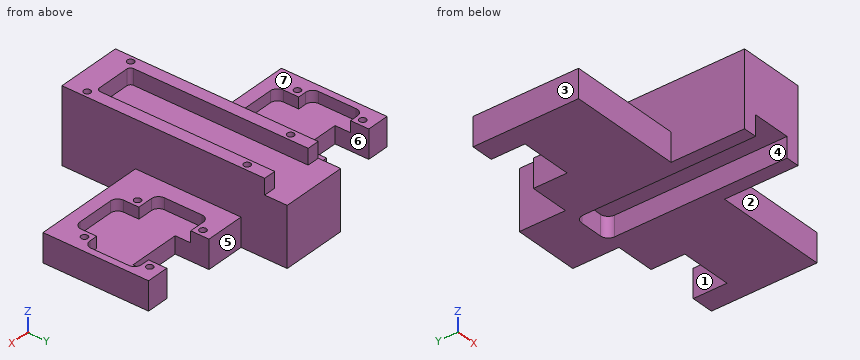
```python
from build123d import *

# Parameters (mm, degrees)
SKETCH1_W           = 130
SKETCH1_H           = 104.86
BOSS_EXTRUDE1_DEPTH = 39.84
SKETCH2_W           = 130
SKETCH2_H           = 94.86
CUT_EXTRUDE1_DEPTH  = 6.6
SKETCH3_W           = 18.25
SKETCH3_H           = 89.15
CUT_EXTRUDE2_DEPTH  = 6.98
SKETCH5_W           = 50.415
SKETCH5_H           = 94.86
CUT_EXTRUDE3_DEPTH  = 20.6
SKETCH6_R           = 1.5
CUT_EXTRUDE4_DEPTH  = 12.4
SKETCH7_W           = 50.415
SKETCH7_H           = 20.5
CUT_EXTRUDE5_DEPTH  = 12.4
SKETCH9_W           = 23
SKETCH9_H           = 15
CUT_EXTRUDE7_DEPTH  = 12.4
CUT_EXTRUDE8_DEPTH  = 5
SKETCH11_R          = 1.5
CUT_EXTRUDE9_DEPTH  = 15
FILLET2_R           = 3.175
FILLET3_R           = 3.175
FILLET4_R           = 3.175
FILLET5_R           = 1.5875
FILLET6_R           = 3.175
SKETCH12_W          = 50.415
SKETCH12_H          = 20.5
SKETCH12_W_2        = 23
SKETCH12_H_2        = 15
SKETCH12_H_3        = 27.5
SKETCH12_W_3        = 29.17
SKETCH12_H_4        = 4.86
CUT_EXTRUDE11_DEPTH = 42
SKETCH13_W          = 6.6
SKETCH13_H          = 5.14
CUT_EXTRUDE12_DEPTH = 80.585
SKETCH14_W          = 29.17
SKETCH14_H          = 10
CUT_EXTRUDE14_DEPTH = 6.98
CUT_EXTRUDE15_DEPTH = 9


with BuildPart() as part:
    # Sketch1 → Boss-Extrude1 (new body)
    with BuildSketch(Plane.XY):
        with Locations((65, -52.43)):
            Rectangle(SKETCH1_W, SKETCH1_H)
    extrude(amount=BOSS_EXTRUDE1_DEPTH)

    # Sketch2 → Cut-Extrude1 (cut)
    with BuildSketch(Plane.XY.offset(39.84)):
        with Locations((65, -47.43)):
            Rectangle(SKETCH2_W, SKETCH2_H)
    extrude(amount=-CUT_EXTRUDE1_DEPTH, mode=Mode.SUBTRACT)

    # Sketch3 → Cut-Extrude2 (cut)
    with BuildSketch(Plane.XY.offset(33.24)):
        with Locations((65, -44.575)):
            Rectangle(SKETCH3_W, SKETCH3_H)
    extrude(amount=-CUT_EXTRUDE2_DEPTH, mode=Mode.SUBTRACT)

    # Sketch5 → Cut-Extrude3 (cut)
    with BuildSketch(Plane.XY.offset(33.24)):
        with Locations((104.7925, -47.43)):
            Rectangle(SKETCH5_W, SKETCH5_H)
        with Locations((25.2075, -47.43)):
            Rectangle(SKETCH5_W, SKETCH5_H)
    extrude(amount=-CUT_EXTRUDE3_DEPTH, mode=Mode.SUBTRACT)

    # Sketch6 → Cut-Extrude4 (cut)
    with BuildSketch(Plane.XY.offset(12.64)):
        with Locations((35.925, -25.6)):
            Circle(SKETCH6_R)
        with Locations((6.925, -25.6)):
            Circle(SKETCH6_R)
        with Locations((35.925, -54.6)):
            Circle(SKETCH6_R)
        with Locations((6.925, -54.6)):
            Circle(SKETCH6_R)
        with Locations((94.075, -25.6)):
            Circle(SKETCH6_R)
        with Locations((123.075, -25.6)):
            Circle(SKETCH6_R)
        with Locations((94.075, -54.6)):
            Circle(SKETCH6_R)
        with Locations((123.075, -54.6)):
            Circle(SKETCH6_R)
    extrude(amount=-CUT_EXTRUDE4_DEPTH, mode=Mode.SUBTRACT)

    # Sketch7 → Cut-Extrude5 (cut)
    with BuildSketch(Plane.XY.offset(12.64)):
        with Locations((25.2075, -10.25)):
            Rectangle(SKETCH7_W, SKETCH7_H)
        with Locations((104.7925, -10.25)):
            Rectangle(SKETCH7_W, SKETCH7_H)
    extrude(amount=-CUT_EXTRUDE5_DEPTH, mode=Mode.SUBTRACT)

    # Sketch9 → Cut-Extrude7 (cut)
    with BuildSketch(Plane.XY.offset(12.64)):
        with Locations((108.575, -28)):
            Rectangle(SKETCH9_W, SKETCH9_H)
        with Locations((21.425, -28)):
            Rectangle(SKETCH9_W, SKETCH9_H)
    extrude(amount=-CUT_EXTRUDE7_DEPTH, mode=Mode.SUBTRACT)

    # Sketch10 → Cut-Extrude8 (cut)
    with BuildSketch(Plane.XY.offset(12.64)):
        Polygon((9.925, -28.6), (3, -28.6), (3, -51.6), (9.925, -51.6), (9.925, -61.6), (32.925, -61.6), (32.925, -51.6), (42.925, -51.6), (42.925, -28.6), (32.925, -28.6), (32.925, -35.5), (9.925, -35.5), align=None)
        Polygon((97.075, -28.6), (87.075, -28.6), (87.075, -51.6), (97.075, -51.6), (97.075, -61.6), (120.075, -61.6), (120.075, -51.6), (127, -51.6), (127, -28.6), (120.075, -28.6), (120.075, -35.5), (97.075, -35.5), align=None)
    extrude(amount=-CUT_EXTRUDE8_DEPTH, mode=Mode.SUBTRACT)

    # Sketch11 → Cut-Extrude9 (cut)
    with BuildSketch(Plane.XY.offset(33.24)):
        with Locations((53.145, -20)):
            Circle(SKETCH11_R)
        with Locations((76.855, -20)):
            Circle(SKETCH11_R)
        with Locations((53.145, -91)):
            Circle(SKETCH11_R)
        with Locations((76.855, -91)):
            Circle(SKETCH11_R)
    extrude(amount=-CUT_EXTRUDE9_DEPTH, mode=Mode.SUBTRACT)

    # Fillet2
    fillet2_edges = [part.edges().sort_by_distance(p)[0] for p in [
        (3, -51.6, 10.14),
    ]]
    fillet(fillet2_edges, radius=FILLET2_R)

    # Fillet3
    fillet3_edges = [part.edges().sort_by_distance(p)[0] for p in [
        (50.415, -20.5, 6.44),
        (79.585, -20.5, 6.44),
        (32.925, -35.5, 3.94),
        (9.925, -35.5, 3.94),
        (42.925, -28.6, 10.14),
        (42.925, -51.6, 10.14),
        (32.925, -61.6, 10.14),
        (9.925, -61.6, 10.14),
        (3, -28.6, 10.14),
        (127, -28.6, 10.14),
        (127, -51.6, 10.14),
        (120.075, -61.6, 10.14),
        (97.075, -61.6, 10.14),
        (87.075, -51.6, 10.14),
        (87.075, -28.6, 10.14),
    ]]
    fillet(fillet3_edges, radius=FILLET3_R)

    # Fillet4
    fillet4_edges = [part.edges().sort_by_distance(p)[0] for p in [
        (120.075, -35.5, 3.94),
        (97.075, -35.5, 3.94),
    ]]
    fillet(fillet4_edges, radius=FILLET4_R)

    # Fillet5
    fillet5_edges = [part.edges().sort_by_distance(p)[0] for p in [
        (74.125, -89.15, 29.75),
        (55.875, -89.15, 29.75),
    ]]
    fillet(fillet5_edges, radius=FILLET5_R)

    # Fillet6
    fillet6_edges = [part.edges().sort_by_distance(p)[0] for p in [
        (79.585, -94.86, 22.94),
        (50.415, -94.86, 22.94),
    ]]
    fillet(fillet6_edges, radius=FILLET6_R)

    # Sketch12 → Cut-Extrude11 (cut)
    with BuildSketch(Plane.XY.offset(39.84)):
        with Locations((25.2075, -10.25)):
            Rectangle(SKETCH12_W, SKETCH12_H)
        with Locations((104.7925, -10.25)):
            Rectangle(SKETCH12_W, SKETCH12_H)
        with Locations((108.575, -28)):
            Rectangle(SKETCH12_W_2, SKETCH12_H_2)
        with Locations((21.425, -28)):
            Rectangle(SKETCH12_W_2, SKETCH12_H_2)
        with Locations((25.2075, -81.11)):
            Rectangle(SKETCH12_W, SKETCH12_H_3)
        with Locations((104.7925, -81.11)):
            Rectangle(SKETCH12_W, SKETCH12_H_3)
        Polygon((130, -94.86), (79.585, -94.86), (79.585, -100), (79.585, -104.86), (130, -104.86), align=None)
        Polygon((50.415, -94.86), (0, -94.86), (0, -104.86), (50.415, -104.86), (50.415, -100), (50.415, -95.14), align=None)
        with Locations((65, -102.43)):
            Rectangle(SKETCH12_W_3, SKETCH12_H_4)
    extrude(amount=-CUT_EXTRUDE11_DEPTH, mode=Mode.SUBTRACT)

    # Sketch13 → Cut-Extrude12 (cut, through all)
    with BuildSketch(Plane(origin=(79.585, 0, 0), x_dir=(0, 0, -1), z_dir=(1, 0, 0))):
        with Locations((-36.54, -97.43)):
            Rectangle(SKETCH13_W, SKETCH13_H)
    extrude(amount=-CUT_EXTRUDE12_DEPTH, mode=Mode.SUBTRACT)

    # Sketch14 → Cut-Extrude14 (cut)
    with BuildSketch(Plane.XY.offset(33.24)):
        with Locations((65, -5)):
            Rectangle(SKETCH14_W, SKETCH14_H)
    extrude(amount=-CUT_EXTRUDE14_DEPTH, mode=Mode.SUBTRACT)

    # Sketch15 → Cut-Extrude15 (cut)
    with BuildSketch(Plane(origin=(0, 0, 0), x_dir=(-1, 0, 0), z_dir=(0, 0, -1))):
        with BuildLine():
            Line((-73.585, -100), (-56.415, -100))
            Line((-56.415, -100), (-56.415, -23.5))
            ThreePointArc((-56.415, -23.5), (-57.440126266, -21.025126266), (-59.915, -20))
            Line((-59.915, -20), (-70.085, -20))
            ThreePointArc((-70.085, -20), (-72.559873734, -21.025126266), (-73.585, -23.5))
            Line((-73.585, -23.5), (-73.585, -100))
        make_face()
    extrude(amount=-CUT_EXTRUDE15_DEPTH, mode=Mode.SUBTRACT)


solid = part.part
```
Geometry check sheet. Reference: the model listing, model coordinates, mm. Face numbers are marked on the shaded views. A direction names the side the tool comes from. Coordinates: 2 decimals unless noted, no trailing zeros. Order: outer loops, then holes, each group sorted by start corner. A loop starts at its lowest first (then second) coordinate and runs counter-clockwise, first axis right, second up. Notation, with made-up numbers: M -23.5,-28.5 L 13.5,-28.5 A26 ccw 13.5,-12.5 Z; hole C 18,19.25 d11. An arc over 180 degrees is marked long. One line per question, with ' | ' between items. Start each with the question number.
Item 1: Set-up check for the marked faces 4, 5, 6 and 7: record each of +Z, -Z, +X, -X, +Y, -Y from which the full face is reachable in a straight line by a thin tool's end or side.
Item 2: Cross-section at D-D on y = -79.5. Enter the section's corners in (x, z) (3 decimals).
Item 3: Cross-section at A-A on y = -34. State how many separate pieces and enclosed holes the cut face has, then the cut area to 3 significant figures.
Item 4: Gauge pin test, flat ends, axial feed: pin 1 (6 mm diameter, centred on y = -17.5, z = 19, fed in from +X) (3 decimals); pin 2 (12 mm diameter, centred on x = 103.5, y = -60, fed in from -Z); pin 3 (4 mm diameter, centred on x = 28, z = 8, fed in from -Y); pin 4 (8 mm diameter, centred on x = 127.5, z = 5, fed in from +Y). Record the tip position at first contact, or that the pin passes through.
Item 5: Cross-section at B-B on z = 23. Enter the section's corners in (x, y) (3 decimals), then the cut area to 3 significant figures.
Item 6: Material ranges on L1, parallel to X at y = -86, z = 28 (3 decimals); L2, parallel to X at y = -79.5, z = 2 (3 decimals); L3, parallel to Y at x = 93.5, z = 7.5, recorded low to high. Write a range as [from, to].
Item 7: Draft check along X on the marked faces 1, 2 and 3. Enter one of: pulls with the +X half, pulls with the -X half, needs draft (parallel to the pull), parting line crosses it, or undercut.
Findings:
1) face 4: -Z, -Y | face 5: +Z, -Z, +X, +Y | face 6: +Z, -Z, +Y | face 7: +Z, -X, +Y, -Y
2) outline: M 50.415,0 L 56.415,0 L 56.415,9 L 73.585,9 L 73.585,0 L 79.585,0 L 79.585,33.24 L 74.125,33.24 L 74.125,26.26 L 55.875,26.26 L 55.875,33.24 L 50.415,33.24 Z
3) separate pieces: 3 | enclosed holes: 0 | area: 1,210 mm²
4) pin 1: stops at x = 79.585 | pin 2: stops at z = 0 | pin 3: stops at y = -67.36 | pin 4: stops at y = -20.5
5) outline: M 50.415,-100 L 79.585,-100 L 79.585,0 L 50.415,0 Z; hole C 53.145,-91 d3; hole C 53.145,-20 d3; hole C 76.855,-91 d3; hole C 76.855,-20 d3 | area: 2,890 mm²
6) L1: x = [50.415, 55.875], [74.125, 79.585] | L2: x = [50.415, 56.415], [73.585, 79.585] | L3: y = [-67.36, -55.99], [-53.21, -26.99], [-24.21, -20.5]
7) face 1: undercut | face 2: needs draft | face 3: pulls with the -X half
